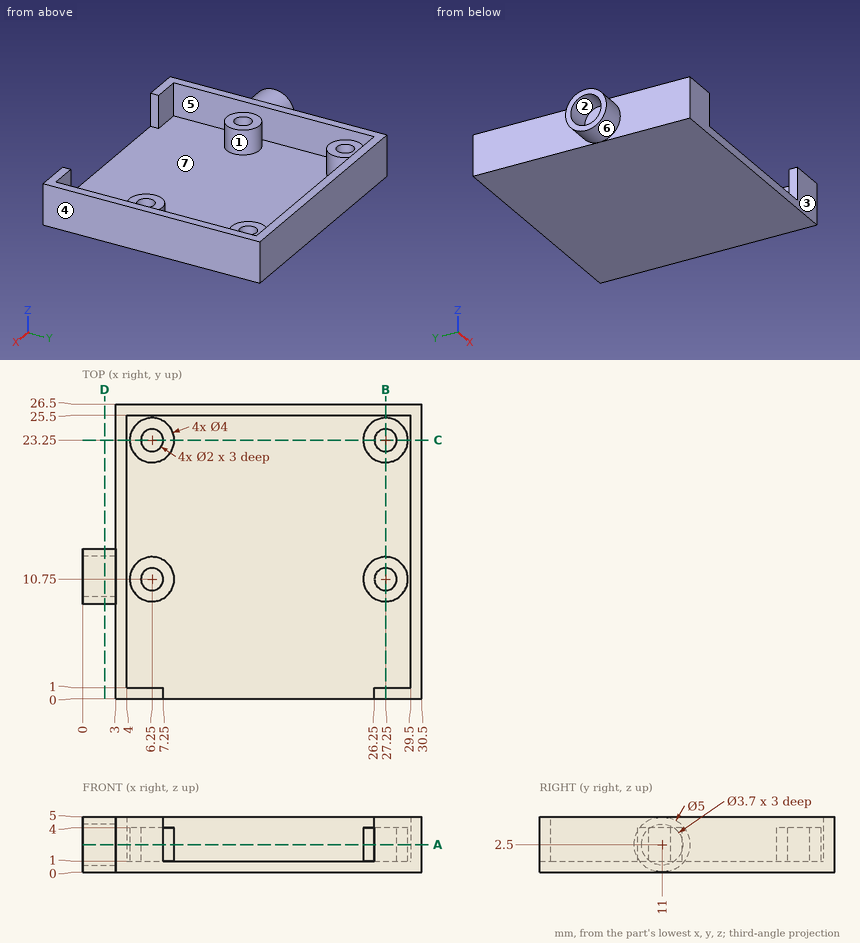
Source: three-view drawing plus pictorial views. Frame: mm from the lowest corner of the part. A direction names the side the tool comes from. Give positions to 0.01 mm unless a question says otherwise; leave off trailing zeros. Write each loop counter-clockwise with the first axis right and the second up, starting at its lowest first coordinate (ties: lowest second). Pieces come first, ordered by that corner, then holes. Notation, with made-up numbers: (43.25, 82) - (102.25, 82) arc R22 ccw to (102.25, 110) - close; hole circle Ø9 at (64, 43). An arc over 180 degrees is marked (long way). Write item = value, one per line. Start each with the question number.
Q1. Cut plane B-B, the plane x = 27.25. Return loops of the section in (y, z), then the cut area to 3 significant figures.
Q2. Cut plane D-D, the plane x = 2. Return loops of the section in (y, z), then the cut area to 3 significant figures.
Q3. Cut plane C-C, the plane y = 23.25. Return loops of the section in (x, z).
Q4. Cut plane A-A, the plane z = 2.5. Give the number of separate pieces and of enclosed holes in the cut face, then the cut area to 3 significant figures.
Q5. Material intervals for probe 1 along Y at (x, z) = (27.25, 3.15); probe 2 along X at (y, z) = (3.25, 3.5); probe 3 along X at (y, z) = (24.75, 1.15), sorted ascending.
Q6. Draft query along Y for the marked faces 4, 5, 6 and 7. Return one class per face: +Y half, -Y half, draft (parallel to the pull), parting line (faces both ways), or undercut.
Q7. Pin query (flat end, axial travel): pin 1 Ø1.2 at (x, y) = (5.5, 23) entering from +Z; pin 2 Ø1.2 at (x, z) = (18, 3) entering from -Y; pin 3 Ø1.2 at (y, z) = (10.5, 2.5) entering from -X. Return the tip coordinate at first contact, or that it passes through.
Q8. Reachability of the marked faces 1, 2 and 3 from +Z, -Z, +X, -X, +Y, -Y: full face, straight path, thin tool, end or side. Return the list, or none.
Computed values:
q1.outline = (0, 0) - (26.5, 0) - (26.5, 5) - (25.5, 5) - (25.5, 1) - (25.25, 1) - (25.25, 4) - (24.25, 4) - (24.25, 1) - (22.25, 1) - (22.25, 4) - (21.25, 4) - (21.25, 1) - (12.75, 1) - (12.75, 4) - (11.75, 4) - (11.75, 1) - (9.75, 1) - (9.75, 4) - (8.75, 4) - (8.75, 1) - (1, 1) - (1, 5) - (0, 5) - close
q1.area = 46.5 mm²
q2.outline = circle Ø5 at (11, 2.5); hole circle Ø3.7 at (11, 2.5)
q2.area = 8.88 mm²
q3.outline = (3, 0) - (30.5, 0) - (30.5, 5) - (29.5, 5) - (29.5, 1) - (29.25, 1) - (29.25, 4) - (28.25, 4) - (28.25, 1) - (26.25, 1) - (26.25, 4) - (25.25, 4) - (25.25, 1) - (8.25, 1) - (8.25, 4) - (7.25, 4) - (7.25, 1) - (5.25, 1) - (5.25, 4) - (4.25, 4) - (4.25, 1) - (4, 1) - (4, 5) - (3, 5) - close
q4.separate_pieces = 5
q4.enclosed_holes = 4
q4.area = 127 mm²
q5.probe_1 = 0 to 1, 8.75 to 9.75, 11.75 to 12.75, 21.25 to 22.25, 24.25 to 25.25, 25.5 to 26.5
q5.probe_2 = 3 to 4, 29.5 to 30.5
q5.probe_3 = 3 to 4, 4.93 to 7.57, 25.93 to 28.57, 29.5 to 30.5
q6.face_4 = draft
q6.face_5 = undercut
q6.face_6 = parting line
q6.face_7 = undercut
q7.pin_1 = 4
q7.pin_2 = 25.5
q7.pin_3 = 3
q8.face_1 = +Z
q8.face_2 = -X
q8.face_3 = +Z, -Z, +X, -X, -Y
